from build123d import *

# Parameters (mm, degrees)
F1_DEPTH = 3.6
F2_R     = 1.1
F3_DEPTH = 8
F4_W     = 2.2
F4_H     = 2
F5_DEPTH = 1.7
F6_R     = 1.6
F7_DEPTH = 1.2
F8_W     = 5.5
F8_H     = 5.5
F9_DEPTH = 2
F10_R    = 0.2


# Not quite as in the source:
# - a feature names something its author has since deleted; it is built from what else it names


with BuildPart() as f1:
    # F0 (on Top) → F1 (new body)
    with BuildSketch(Plane.XY):
        Polygon((30, 15), (-30, 15), (-30, 9.6), (-5.6, 9.6), (-5.6, -15), (5.6, -15), (5.6, 9.6), (30, 9.6), align=None)
    extrude(amount=F1_DEPTH)

    # F2 (on face) → F3 (cut)
    with BuildSketch(Plane.XZ.offset(15)):
        with Locations((0, 1.9)):
            Circle(F2_R)
    extrude(amount=-F3_DEPTH, mode=Mode.SUBTRACT)

    # F4 (on face) → F5 (cut)
    with BuildSketch(Plane.XY.offset(3.6)):
        with Locations((0, -14)):
            Rectangle(F4_W, F4_H)
        with BuildLine():
            ThreePointArc((1.1, -13), (0, -11.9), (-1.1, -13))
            Line((-1.1, -13), (1.1, -13))
        make_face()
    extrude(amount=-F5_DEPTH, mode=Mode.SUBTRACT)

    # F6 (on face) → F7 (cut)
    with BuildSketch(Plane(origin=(0, 0, 0), x_dir=(1, 0, 0), z_dir=(0, 0, -1))):
        with Locations((0, 5)):
            Circle(F6_R)
        with Locations((0, -3.3)):
            Circle(F6_R)
        with Locations((25, -12.3)):
            Circle(F6_R)
        with Locations((-25, -12.3)):
            Circle(F6_R)
        with Locations((0, -12.3)):
            Circle(F6_R)
    extrude(amount=-F7_DEPTH, mode=Mode.SUBTRACT)

    # F8 (on face) → F9 (cut)
    with BuildSketch(Plane.XY.offset(3.6)):
        with Locations((0, -2.25)):
            Rectangle(F8_W, F8_H)
    extrude(amount=-F9_DEPTH, mode=Mode.SUBTRACT)

    # F10
    f10_edges = [f1.edges().sort_by_distance(p)[0] for p in [
        (-5.6, 9.6, 1.8),
        (5.6, 9.6, 1.8),
        (30, 15, 1.8),
        (-30, 15, 1.8),
        (-2.75, 0.5, 2.6),
        (2.75, 0.5, 2.6),
        (2.75, -5, 2.6),
        (-2.75, -5, 2.6),
        (5.6, -15, 1.8),
        (-5.6, -15, 1.8),
    ]]
    fillet(f10_edges, radius=F10_R)


solid = f1.part
Read the model definition and answer for the solid it produces. Units are mm, in the model's axes. A direction names the side the tool comes from. Give positions to 0.01 mm unless a question says otherwise; leave off trailing zeros. Write each loop counter-clockwise with the first axis right and the second up, starting at its lowest first coordinate (ties: lowest second). Pieces come first, ordered by that corner, then holes. Notation, with made-up numbers: (82.25, -26.75) -> (119.25, -26.75) arc R22 ccw to (119.25, 11.25) -> close; hole circle Ø11 at (22.25, 11). An arc over 180 degrees is marked (long way). Answer as a JSON object with one key per item and string values. Group by question number.
1) The mould has two halves that part along Y. Classify faces 1 (the flat face through (0, 0.5, 3)), 2 (the flat face through (1.1, -14, 3)), 3 (the flat face through (0, -2, 1.6)), 4 (the cylindrical face through (0, -11.9, 3.3)): +Y half, -Y half, draft (parallel to the pull), parting line (faces both ways), or undercut.
2) Consider L1, parallel to Y at x = 0, z = 1.05; L2, parallel to X at y = 12.3, z = 0.9; L3, parallel to X at y = -5, z = 0.65. Determine where each line is inside the solid, lowest interval first. Write a range as from..to.
3) Find section C-C (y = -8). Write down the section's boundary in (x, z), and give its area (3 significant figures).
4) Find section A-A (y = 3.3). Write down the section's boundary in (x, z).
5) Find section D-D (y = 12.3). Write down the section's boundary in (x, z), and give its area (3 significant figures).
6) Each of these flat-tipped pins is pushed along its axis until it touches: P1, Ø1.4, axis at y = -14, z = 3, coming from the +X side; P2, Ø1.1, axis at x = -0.5, z = 2, coming from the -Y side; P3, Ø0.6, axis at y = -1.5, z = 2.5, coming from the -X side. Where does it stop, or does it pass through?
7) Find section B-B (x = 25). Write down the section's boundary in (y, z), and give its area (3 significant figures).
8) A tool of negligible diameter and unlimited length cuts with its end or side. For faces 5 (the flat face through (18, 9.6, 2)), 6 (the flat face through (-18, 9.6, 2)), 7 (the flat face through (-1.1, -14, 3)), 8 (the flat face through (25, 12, 1.2)), 9 (the flat face through (0, -5, 3)), from which of +Z, -Z, +X, -X, +Y, -Y can it reach the whole face along a straight path? Write none if from no direction.
Values follow:
{
 "1": {"face 1": "undercut", "face 2": "draft", "face 3": "undercut", "face 4": "-Y half"},
 "2": {"L1": "y = -7..-6.6, -3.4..1.7, 4.9..10.7, 13.9..15", "L2": "x = -30..-26.6, -23.4..-1.6, 1.6..23.4, 26.6..30", "L3": "x = -5.6..-1.6, 1.6..5.6"},
 "3": {"outline": "(-5.6, 0) -> (5.6, 0) -> (5.6, 3.6) -> (-5.6, 3.6) -> close; hole circle Ø2.2 at (0, 1.9)", "area": "36.5 mm2"},
 "4": {"outline": "(-5.6, 0) -> (-1.6, 0) -> (-1.6, 1.2) -> (1.6, 1.2) -> (1.6, 0) -> (5.6, 0) -> (5.6, 3.6) -> (-5.6, 3.6) -> close"},
 "5": {"outline": "(-30, 0) -> (-26.6, 0) -> (-26.6, 1.2) -> (-23.4, 1.2) -> (-23.4, 0) -> (-1.6, 0) -> (-1.6, 1.2) -> (1.6, 1.2) -> (1.6, 0) -> (23.4, 0) -> (23.4, 1.2) -> (26.6, 1.2) -> (26.6, 0) -> (30, 0) -> (30, 3.6) -> (-30, 3.6) -> close", "area": "204 mm2"},
 "6": {"P1": "stops at x = 5.6", "P2": "stops at y = -7", "P3": "stops at x = -5.6"},
 "7": {"outline": "(9.6, 0) -> (10.7, 0) -> (10.7, 1.2) -> (13.9, 1.2) -> (13.9, 0) -> (15, 0) -> (15, 3.6) -> (9.6, 3.6) -> close", "area": "15.6 mm2"},
 "8": {"face 5": "+Z, -Z, +X, -Y", "face 6": "+Z, -Z, -X, -Y", "face 7": "+Z, -Y", "face 8": "-Z", "face 9": "+Z"}
}
